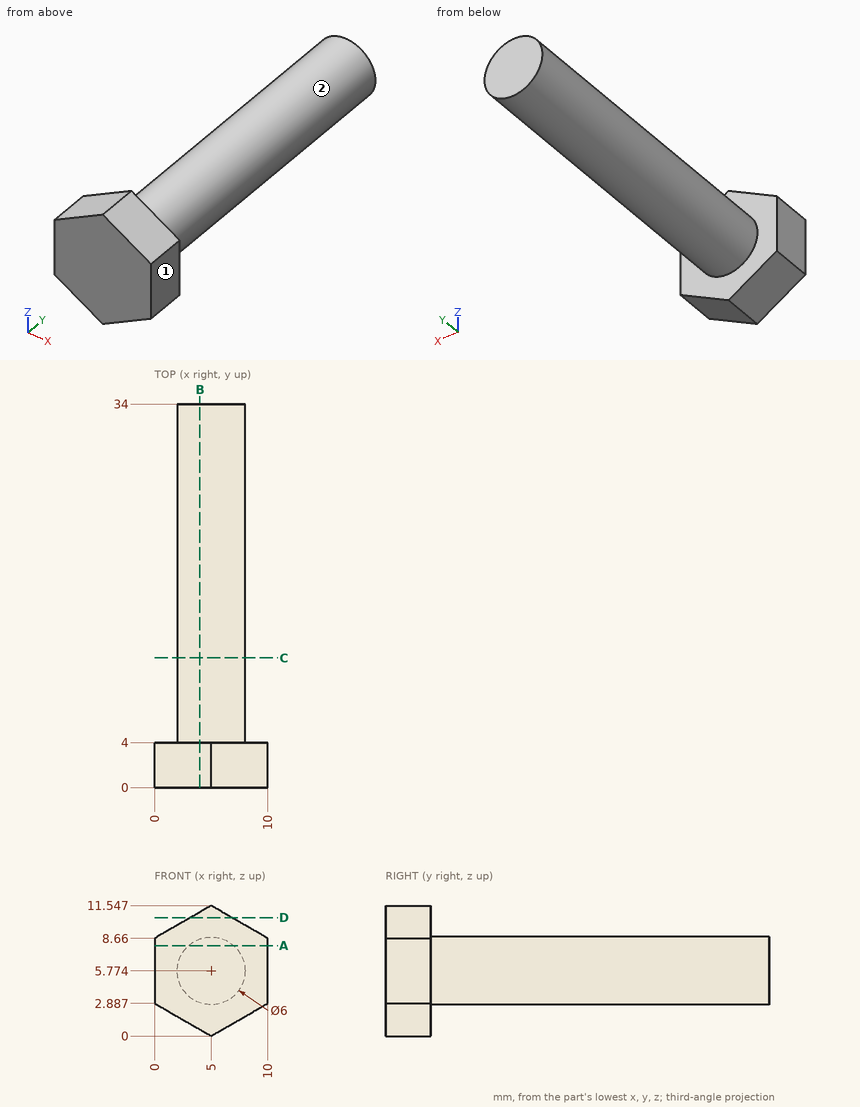
Check sheet for the drawn part. Datum: minimum x, y, z corner. Units: mm. A direction names the side the tool comes from. Give positions to 0.01 mm unless a question says otherwise; leave off trailing zeros. Order: outer loops, then holes, each group sorted by start corner. A loop starts at its lowest first (then second) coordinate and runs counter-clockwise, first axis right, second up. Notation, with made-up numbers: (72.5, 75.25) - (123.5, 75.25) arc R13 cw to (123.5, 80.25) - close; hole circle Ø2 at (-23, 26). An arc over 180 degrees is marked (long way). Write item = value, one per line. Start each with the question number.
1) Section check A-A (z = 8). Enter the section's corners in (x, y), then the cut area to 3 significant figures.
2) Scan lines: L1, parallel to Y at x = 2, z = 8; L2, parallel to X at y = 6.5, z = 5.75; L3, parallel to Z at x = 7.5, y = 3 (1 decimal). Record each from-to range of solid material in increasing order.
3) Access from +Z, -Z, +X, -X, +Y, -Y to the whole of each face (thin tool, end or side, straight path). Record for the marked faces 1 and 2.
4) Section check B-B (x = 4). Enter the section's corners in (y, z) (1 decimal), then the cut area to 3 significant figures.
5) Gauge pin test, flat ends, axial feed: pin 1 Ø3 at (y, z) = (11, 1.5) entering from +X (1 decimal); pin 2 Ø1 at (x, y) = (1, 11.5) entering from +Z; pin 3 Ø1 at (x, y) = (4.5, 12.5) entering from +Z. Record the tip position at first contact, or that the pin passes through.
6) Section check C-C (y = 11.5). Enter the section's corners in (x, z), then the cut area to 3 significant figures.
7) Section check D-D (z = 10.5). Enter the section's corners in (x, y).
Geometry check:
q1.outline = (0, 0) - (10, 0) - (10, 4) - (7.01, 4) - (7.01, 34) - (2.99, 34) - (2.99, 4) - (0, 4) - close
q1.area = 161 mm2
q2.L1 = 0 to 4
q2.L2 = 2 to 8
q2.L3 = 1.4 to 10.1
q3.face_1 = +Z, -Z, +X, +Y, -Y
q3.face_2 = +Y
q4.outline = (0, 0.6) - (4, 0.6) - (4, 2.9) - (34, 2.9) - (34, 8.6) - (4, 8.6) - (4, 11) - (0, 11) - close
q4.area = 211 mm2
q5.pin_1 = 6.1
q5.pin_2 = through
q5.pin_3 = 8.77
q6.outline = circle Ø6 at (5, 5.77)
q6.area = 28.3 mm2
q7.outline = (3.19, 0) - (6.81, 0) - (6.81, 4) - (3.19, 4) - close
